Check sheet for the modelled part. Datum: model origin and axes. Units: mm. A direction names the side the tool comes from. Round coordinates to 2 decimals unless told otherwise and drop trailing zeros. Loops run counter-clockwise (first coordinate to the right, second up) from the corner with the lowest first, then second, coordinate; pieces in that order, holes last. Notation, with made-up numbers: (11.25, 84) - (60.25, 84) arc R29 ccw to (60.25, 105) - close; hole circle Ø8 at (16.5, -3). An arc over 180 degrees is marked (long way). Return JSON: item names as keys, results as strings.
from build123d import *

# Parameters (mm, degrees)
SKETCH012_R         = 1.2
SKETCH012_W         = 12
SKETCH012_H         = 7
SKETCH012_H_2       = 3
PAD006_DEPTH        = 1.8
CHAMFER002_ANGLE    = 45
CHAMFER002_SIZE     = 0.9
POCKET_DEPTH        = 1.801
LINEARPATTERN_COUNT = 5
LINEARPATTERN_PITCH = 6
SKETCH015_W         = 16
SKETCH015_H         = 20.8
SKETCH015_W_2       = 12
SKETCH015_H_2       = 16.6
PAD007_DEPTH        = 6
SKETCH016_R         = 1.3
PAD008_DEPTH        = 4
SKETCH017_R         = 0.7
POCKET007_DEPTH     = 4
SKETCH018_W         = 14
SKETCH018_H         = 18.8
POCKET008_DEPTH     = 1


with BuildPart() as part:
    # Sketch012 → Pad006 (new body)
    with BuildSketch(Plane.XY.offset(56)):
        with BuildLine():
            Line((-29.2, -1), (29.2, -1))
            Line((29.2, -1), (29.2, -42))
            add(Edge.make_bspline(
                [(24.4, -42), (24.4, -46), (26.8, -46), (29.2, -46), (29.2, -42)],
                knots=[4.712389, 4.712389, 4.712389, 6.283185, 6.283185, 7.853982, 7.853982, 7.853982], degree=2, weights=[1, 0.707107, 1, 0.707107, 1]))
            Line((24.4, -42), (-24.4, -42))
            add(Edge.make_bspline(
                [(-29.2, -42), (-29.2, -46), (-26.8, -46), (-24.4, -46), (-24.4, -42)],
                knots=[4.712389, 4.712389, 4.712389, 6.283185, 6.283185, 7.853982, 7.853982, 7.853982], degree=2, weights=[1, 0.707107, 1, 0.707107, 1]))
            Line((-29.2, -42), (-29.2, -1))
        make_face()
        with Locations((-26.9, -43.8)):
            Circle(SKETCH012_R, mode=Mode.SUBTRACT)
        with Locations((26.9, -43.8)):
            Circle(SKETCH012_R, mode=Mode.SUBTRACT)
        with Locations((-12.5, -36.7)):
            Rectangle(SKETCH012_W, SKETCH012_H, mode=Mode.SUBTRACT)
        with Locations((-12.5, -21.5)):
            Rectangle(SKETCH012_W, SKETCH012_H_2, mode=Mode.SUBTRACT)
    extrude(amount=PAD006_DEPTH)

    # Chamfer002
    chamfer002_edges = [part.edges().sort_by_distance(p)[0] for p in [
        (0, -1, 57.8),
    ]]
    chamfer002_side = part.faces().sort_by_distance((0, -1, 56.9))[0]
    chamfer(chamfer002_edges, length=CHAMFER002_SIZE, angle=CHAMFER002_ANGLE, reference=chamfer002_side)

    # Sketch013 → Pocket (cut, through all)
    with BuildSketch(Plane.XY.offset(57.8)):
        Polygon((7.827629, -35.616149), (9.027629, -33.537688), (7.827629, -31.459227), (5.427629, -31.459227), (4.227629, -33.537688), (5.427629, -35.616149), align=None)
        Polygon((19.184551, -35.616149), (20.384551, -33.537688), (19.184551, -31.459227), (16.784551, -31.459227), (15.584551, -33.537688), (16.784551, -35.616149), align=None)
        Polygon((13.50609, -38.89461), (14.70609, -36.816149), (13.50609, -34.737688), (11.10609, -34.737688), (9.90609, -36.816149), (11.10609, -38.89461), align=None)
        Polygon((24.863012, -38.89461), (26.063012, -36.816149), (24.863012, -34.737688), (22.463012, -34.737688), (21.263012, -36.816149), (22.463012, -38.89461), align=None)
    pocket = extrude(amount=-POCKET_DEPTH, mode=Mode.SUBTRACT)

    # LinearPattern: Pocket ×5
    with Locations(*[(0, i * LINEARPATTERN_PITCH, 0) for i in range(1, LINEARPATTERN_COUNT)]):
        add(pocket, mode=Mode.SUBTRACT)

    # Sketch015 (on DatumPlane) → Pad007 (join)
    with BuildSketch(Plane.XY.offset(57.8)):
        with Locations((-12.5, -14.6)):
            Rectangle(SKETCH015_W, SKETCH015_H)
        with Locations((-12.5, -14.7)):
            Rectangle(SKETCH015_W_2, SKETCH015_H_2, mode=Mode.SUBTRACT)
    extrude(amount=PAD007_DEPTH)

    # Sketch016 (on DatumPlane) → Pad008 (join)
    with BuildSketch(Plane.XY.offset(57.8)):
        with Locations((-9.9, -11.6)):
            Circle(SKETCH016_R)
    extrude(amount=PAD008_DEPTH)

    # Sketch017 (on Face156 of Pocket008) → Pocket007 (cut)
    with BuildSketch(Plane.XY.offset(61.8)):
        with Locations((-9.9, -11.6)):
            Circle(SKETCH017_R)
    extrude(amount=-POCKET007_DEPTH, mode=Mode.SUBTRACT)

    # Sketch018 (on Face148 of Pocket007) → Pocket008 (cut)
    with BuildSketch(Plane.XY.offset(63.8)):
        with Locations((-12.5, -14.6)):
            Rectangle(SKETCH018_W, SKETCH018_H)
    extrude(amount=-POCKET008_DEPTH, mode=Mode.SUBTRACT)


solid = part.part
Q1. Draft check along Y on faces 1 (the face through (7, -31.459, 57)), 2 (the face through (0, -18, 56)). Enter one of: released by +Y, released by -Y, zero draft, split by the parting line, or undercut.
Answer key:
{"face 1": "undercut", "face 2": "zero draft"}
Q2. Sectioned sample at A-A (z = 60). Enter the section's corners in (x, y), plus the area to 3 significant figures.
Answer key:
{"outline": "(-20.5, -25) - (-4.5, -25) - (-4.5, -4.2) - (-20.5, -4.2) - close; circle Ø2.6 at (-9.9, -11.6); hole (-18.5, -23) - (-6.5, -23) - (-6.5, -6.4) - (-18.5, -6.4) - close; hole circle Ø1.4 at (-9.9, -11.6)", "area": "137 mm²"}
Q3. Scan lines: probe 1 along Y at (x, z) = (-9.9, 60.8); probe 2 along X at (y, z) = (-21, 56.5); probe 3 along X at (y, z) = (-22.5, 63.75). Record each from-to range of solid material in increasing order. Write a range as [from, to].
Answer key:
{"probe 1": "y = [-25, -23], [-12.9, -12.3], [-10.9, -10.3], [-6.4, -4.2]", "probe 2": "x = [-29.2, -18.5], [-6.5, 4.54], [8.72, 15.89], [20.07, 29.2]", "probe 3": "x = [-20.5, -19.5], [-5.5, -4.5]"}
Q4. Sectioned sample at B-B (y = -43.8). State how many separate pieces and enclosed holes the cut face has, plus the area to 3 significant figures.
Answer key:
{"separate pieces": "4", "enclosed holes": "0", "area": "6.79 mm²"}
Q5. Tool access check on faces 3 (the face through (-13, -33.2, 57)), 4 (the face through (-6.5, -15, 60)). Record the directions out of +Z, -Z, +X, -X, +Y, -Y that give a thin tool (end or side, any length) a straight path to the whole face; none if there is none.
Answer key:
{"face 3": "+Z, -Z", "face 4": "+Z"}
Q6. Depth check by flat-ended pin: P1, Ø0.5, axis at x = -11, z = 56.5, coming from the -Y side; P2, Ø4, axis at y = -12.5, z = 60.5, coming from the +X side; P3, Ø2, axis at x = 5, y = -11, coming from the +Z side. Enter the tip coordinate at first touch or a pass-through.
Answer key:
{"P1": "stops at y = -42", "P2": "stops at x = -4.5", "P3": "stops at z = 57.8"}
